```python
from build123d import *

# Parameters (mm, degrees)
SKETCH_1_W          = 40
SKETCH_1_H          = 120
EXTRUDE_1_DEPTH     = 12
EXTRUDE_2_DEPTH     = 40
SKETCH_3_R          = 17.5
CUT_EXTRUDE_1_DEPTH = 121
CUT_EXTRUDE_2_DEPTH = 90.269255626


with BuildPart() as part:
    # 草图1 → 凸台-拉伸1 (new body)
    with BuildSketch(Plane(origin=(0, 0, 0), x_dir=(1, 0, 0), z_dir=(0, 1, 0))):
        Rectangle(SKETCH_1_W, SKETCH_1_H)
    extrude(amount=EXTRUDE_1_DEPTH)

    # 草图2 → 凸台-拉伸2 (add)
    with BuildSketch(Plane(origin=(-20, 0, 0), x_dir=(0, 0, -1), z_dir=(1, 0, 0))):
        with BuildLine():
            Line((30, 10), (30, 45))
            ThreePointArc((30, 45), (0, 75), (-30, 45))
            Line((-30, 45), (-30, 10))
            Line((-30, 10), (30, 10))
        make_face()
    extrude(amount=EXTRUDE_2_DEPTH)

    # 草图3 → 切除-拉伸1 (cut, symmetric)
    with BuildSketch(Plane(origin=(0, 0, 0), x_dir=(0, 0, -1), z_dir=(1, 0, 0))):
        with Locations((0, 45)):
            Circle(SKETCH_3_R)
    extrude(amount=CUT_EXTRUDE_1_DEPTH, both=True, mode=Mode.SUBTRACT)

    # 草图4 → 切除-拉伸2 (cut, through all)
    with BuildSketch(Plane(origin=(0, 12, 0), x_dir=(1, 0, 0), z_dir=(0, 1, 0))):
        with BuildLine():
            Line((5.5, -40), (5.5, -50))
            ThreePointArc((5.5, -50), (0, -55.5), (-5.5, -50))
            Line((-5.5, -50), (-5.5, -40))
            ThreePointArc((-5.5, -40), (0, -34.5), (5.5, -40))
        make_face()
        with BuildLine():
            Line((5.5, 50), (5.5, 40))
            ThreePointArc((5.5, 40), (0, 34.5), (-5.5, 40))
            Line((-5.5, 40), (-5.5, 50))
            ThreePointArc((-5.5, 50), (0, 55.5), (5.5, 50))
        make_face()
    extrude(amount=-CUT_EXTRUDE_2_DEPTH, mode=Mode.SUBTRACT)


solid = part.part
```
The model under review builds one solid part; all positions refer to its coordinate system, in mm. A direction names the side the tool comes from. Coordinates: 2 decimals unless noted, no trailing zeros. Write each loop counter-clockwise with the first axis right and the second up, starting at its lowest first coordinate (ties: lowest second). Pieces come first, ordered by that corner, then holes. Notation, with made-up numbers: (78, -3.75) - (132, -3.75) arc R24 cw to (132, 7.25) - close; hole circle Ø7 at (44.5, 80). An arc over 180 degrees is marked (long way). Write item = value, one per line.
(1) Consider section C-C, the plane z = 0. Give the boundary of the cut face in (x, y), then the cut area to 3 significant figures.
Result sheet:
outline = (-20, 0) - (20, 0) - (20, 27.5) - (-20, 27.5) - close; (-20, 62.5) - (20, 62.5) - (20, 75) - (-20, 75) - close
area = 1,600 mm^2
(2) For line 1 (Y direction, x = 11.5, z = 0); line 2 (Z direction, x = 11.5, y = 14.5); line 3 (Y direction, x = -5.5, z = 31.5), list the stretches that pass through material, from the lowest coordinate up. Write a range as [from, to].
Result sheet:
line_1 = [0, 27.5], [62.5, 75]
line_2 = [-30, 30]
line_3 = [0, 12]
(3) Machinability: for faces 4 (the face through (0, 28, -30)), 5 (the face through (0.1, 6.1, -34.5)), 6 (the face through (-9, 12, 45)), which of the approach directions +Z, -Z, +X, -X, +Y, -Y give a long, thin tool a straight path to every point of the face, cutting with its end or side? Answer none if there is none.
Result sheet:
face_4 = -Z, +X, -X, +Y
face_5 = +Y, -Y
face_6 = +Z, +X, -X, +Y
(4) Consider section B-B, the plane x = 17.5. Give the boundary of the cut face in (y, z), then the cut area to 3 significant figures.
Result sheet:
outline = (0, -60) - (12, -60) - (12, -30) - (45, -30) arc R30 ccw to (45, 30) - (12, 30) - (12, 60) - (0, 60) - close; hole circle Ø35 at (45, 0)
area = 3,870 mm^2
(5) Consider section D-D, the plane y = 58. Give the boundary of the cut face in (x, z).
Result sheet:
outline = (-20, -27.04) - (20, -27.04) - (20, -11.72) - (-20, -11.72) - close; (-20, 11.72) - (20, 11.72) - (20, 27.04) - (-20, 27.04) - close
(6) Consider section A-A, the plane x = 0. Give the boundary of the cut face in (y, z), then the cut area to 3 significant figures.
Result sheet:
outline = (0, -60) - (12, -60) - (12, -55.5) - (0, -55.5) - close; (0, -34.5) - (12, -34.5) - (12, -30) - (45, -30) arc R30 ccw to (45, 30) - (12, 30) - (12, 34.5) - (0, 34.5) - close; (0, 55.5) - (12, 55.5) - (12, 60) - (0, 60) - close; hole circle Ø35 at (45, 0)
area = 3,370 mm^2
(7) For P1, Ø9, axis at x = 2, z = -49.5, coming from the +Y side; P2, Ø16.5, axis at x = 9, y = 20.5, coming from the -Z side; P3, Ø5, axis at x = -6, y = 41, coming from the +Z side, all flat-tipped, find the tip position at first contact; note any pin that passes through.
Result sheet:
P1 = 12
P2 = -30
P3 = 30
(8) Mouldability with a two-part tool opening along X and no side actions: class faces 1 (the face through (-0.1, 6.1, -55.5)), 2 (the face through (0, 0, -1)), 3 (the face through (20, 20, 1)) as pulls with the +X half, pulls with the -X half, needs draft (parallel to the pull), parting line crosses it, or undercut.
Result sheet:
face_1 = undercut
face_2 = needs draft
face_3 = pulls with the +X half
